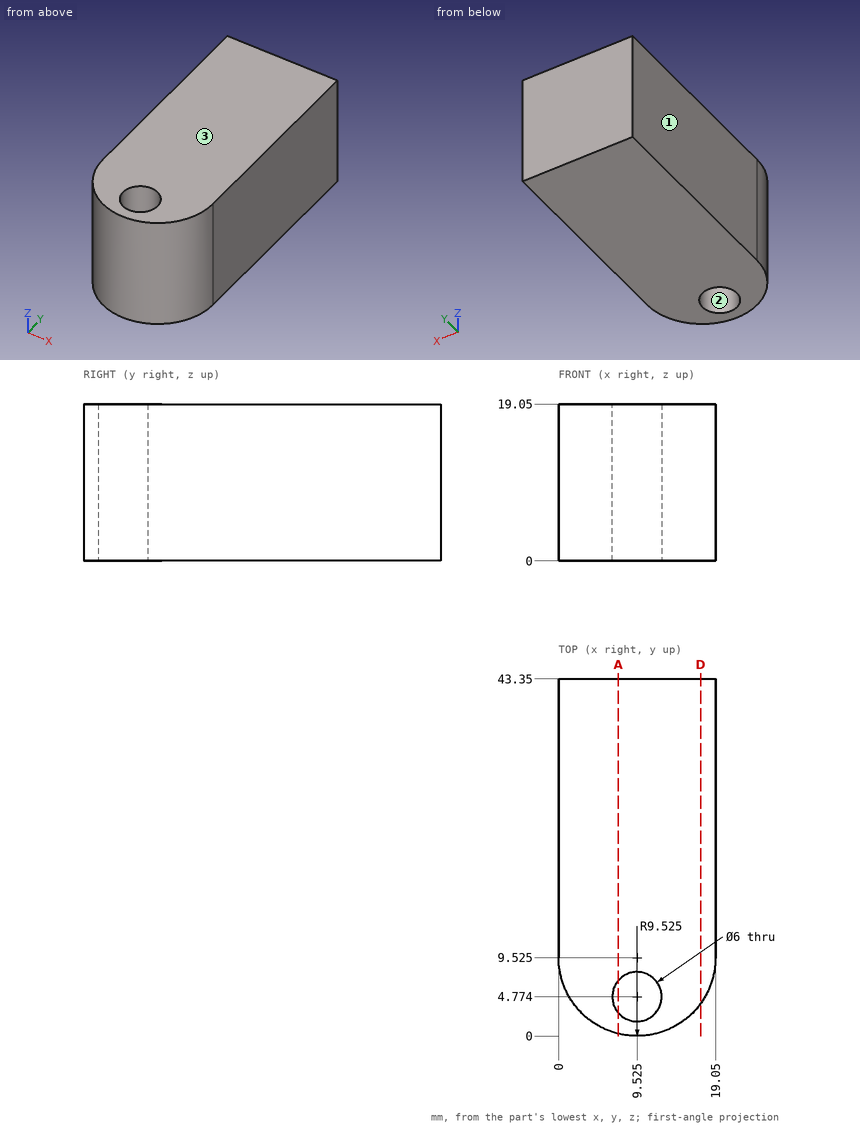
Study the drawing (mm; zero at the part's minimum x, y, z) and answer. Coordinates: 2 decimals unless noted, no trailing zeros. Write each loop counter-clockwise with the first axis right and the second up, starting at its lowest first coordinate (ties: lowest second). Pieces come first, ordered by that corner, then holes. Notation, with made-up numbers: (69.5, 4) - (120.5, 4) arc R20 ccw to (120.5, 32) - close; hole circle Ø9 at (-4, -40). An arc over 180 degrees is marked (long way). Put each result on its own line as item: value.
1. Determine the mould class of the marked faces 1, 2 and 3 for opening direction X: pulls with the +X half, pulls with the -X half, needs draft (parallel to the pull), parting line crosses it, or undercut.
Answer sheet:
face 1: pulls with the -X half
face 2: undercut
face 3: needs draft
2. A flat-ended cylindrical pin translates along its axis: pin 1 Ø5.5 at (x, y) = (9.52, 4.77) entering from -Z. Find the tip coordinate at first contact, or state that the pin passes through.
Answer sheet:
pin 1: passes through
3. Find the intervals of material crossed by line 1 along Y through (x, z) = (8, 8); line 2 along Y through (x, z) = (7.5, 16.25); line 3 along Y through (x, z) = (15.25, 10.5), in increasing order. Write a range as from..to.
Answer sheet:
line 1: y = 0.12..2.19, 7.36..43.35
line 2: y = 0.22..2.56, 6.99..43.35
line 3: y = 1.91..43.35
4. The part is cut by section D-D on x = 17.25. Give the vertices of the cut face in (y, z).
Answer sheet:
outline: (3.95, 0) - (43.35, 0) - (43.35, 19.05) - (3.95, 19.05) - close
5. The part is cut by section A-A on x = 7.25. Give the vertices of the cut face in (y, z).
Answer sheet:
outline: (0.28, 0) - (2.82, 0) - (2.82, 19.05) - (0.28, 19.05) - close; (6.73, 0) - (43.35, 0) - (43.35, 19.05) - (6.73, 19.05) - close
